Work out the finished part from the listing and answer in its coordinate system (mm). A direction names the side the tool comes from. Round coordinates to 2 decimals unless told otherwise and drop trailing zeros. Order: outer loops, then holes, each group sorted by start corner. A loop starts at its lowest first (then second) coordinate and runs counter-clockwise, first axis right, second up. Notation, with made-up numbers: (-27.75, 32.25) - (-17.75, 32.25) arc R37 cw to (-17.75, 70.25) - close; hole circle Ø7 at (74.5, 33.5). An arc over 180 degrees is marked (long way). Use CSV: the item, a comma, the result in double quotes.
Solid Edge part; units mm, degrees
sketch "Sketch1" plane through (0, 0, 0) normal (0, 0, 1) x (1, 0, 0)
  circle A0 centre (0, 0) radius 31.5
extrude "Protrusion1" add sketch "Sketch1" along normal blind 10
hole "Hole_1" at (-17.6777, 17.6777, 10) direction (0, 0, -1) diameter 6.6 end up to next counterbore diameter 11 counterbore depth 6.4
hole "Hole1" at (17.6777, 17.6777, 10) direction (0, 0, -1) diameter 6.6 end up to next counterbore diameter 11 counterbore depth 6.4
hole "Hole2" at (-17.6777, -17.6777, 10) direction (0, 0, -1) diameter 6.6 end up to next counterbore diameter 11 counterbore depth 6.4
hole "Hole3" at (17.6777, -17.6777, 10) direction (0, 0, -1) diameter 6.6 end up to next counterbore diameter 11 counterbore depth 6.4
hole "Hole4" at (0, 25, 10) direction (0, 0, -1) diameter 6 end up to next
hole "Hole_6" at (-20.5, 0, 10) direction (0, 0, -1) diameter 4 end up to next thread major 4 thread length 2
hole "Hole5" at (20.5, 0, 10) direction (0, 0, -1) diameter 4 end up to next thread major 4 thread length 2
(1) Find section B-B (y = 25). Determine the outline of the cut face in (x, z).
Findings below:
outline,"(-19.16, 0) - (-3, 0) - (-3, 10) - (-19.16, 10) - close; (3, 0) - (19.16, 0) - (19.16, 10) - (3, 10) - close"
(2) Each of these flat-tipped pins is pushed along its axis until it touches: pin 1 (1 mm diameter, centred on y = -11.5, z = 5, fed in from +X); pin 2 (5 mm diameter, centred on y = -24, z = 7.5, fed in from -X); pin 3 (1 mm diameter, centred on x = 17, z = 6.5, fed in from -Y). Where does it stop, or does it pass through?
Findings below:
pin 1,"stops at x = 29.52"
pin 2,"stops at x = -23.02"
pin 3,"stops at y = -26.83"
(3) Find section C-C (y = 0). Determine the outline of the cut face in (x, z), and give its area (3 significant figures).
Findings below:
outline,"(-31.5, 0) - (-22.5, 0) - (-22.5, 10) - (-31.5, 10) - close; (-18.5, 0) - (18.5, 0) - (18.5, 10) - (-18.5, 10) - close; (22.5, 0) - (31.5, 0) - (31.5, 10) - (22.5, 10) - close"
area,"550 mm²"
(4) Find section A-A (x = 0). Determine the outline of the cut face in (y, z), and give its area (3 significant figures).
Findings below:
outline,"(-31.5, 0) - (22, 0) - (22, 10) - (-31.5, 10) - close; (28, 0) - (31.5, 0) - (31.5, 10) - (28, 10) - close"
area,"570 mm²"
(5) Find section D-D (z = 1.75). Determine the outline of the cut face in (x, y), and give its area (3 significant figures).
Findings below:
outline,"circle Ø63 at (0, 0); hole circle Ø4 at (-20.5, 0); hole circle Ø6.6 at (-17.68, -17.68); hole circle Ø6.6 at (-17.68, 17.68); hole circle Ø6 at (0, 25); hole circle Ø6.6 at (17.68, -17.68); hole circle Ø6.6 at (17.68, 17.68); hole circle Ø4 at (20.5, 0)"
area,"2,930 mm²"
(6) Find the intervals of material crossed by L1, parallel to X at y = -20, z = 1; L2, parallel to X at y = 21.5, z = 5.25; L3, parallel to Y at x = 2.5, z = 7, in increasing order. Write a range as from..to.
Findings below:
L1,"x = -24.34..-20.02, -15.33..15.33, 20.02..24.34"
L2,"x = -23.02..-21.63, -13.72..13.72, 21.63..23.02"
L3,"y = -31.4..23.34, 26.66..31.4"
(7) The mould has two halves that part along X. Classify faces 3 (the cylindrical face through (-19.69, -15.06, 1.83)), 4 (the flat face through (0, 0, 0)), 5 (the cylindrical face through (-4.101, -31.232, 4.93)): released by +X, released by -X, zero draft, split by the parting line, or undercut.
Findings below:
face 3,"undercut"
face 4,"zero draft"
face 5,"split by the parting line"
(8) For faces 1 (the cylindrical face through (-17.92, 23.172, 6.755)), 2 (the cylindrical face through (22.483, 0.26, 5.07)), determine the directions among +Z, -Z, +X, -X, +Y, -Y from which every point of the face is accessible in a straight line to the end or side of a thin tool.
Findings below:
face 1,"+Z"
face 2,"+Z, -Z"
